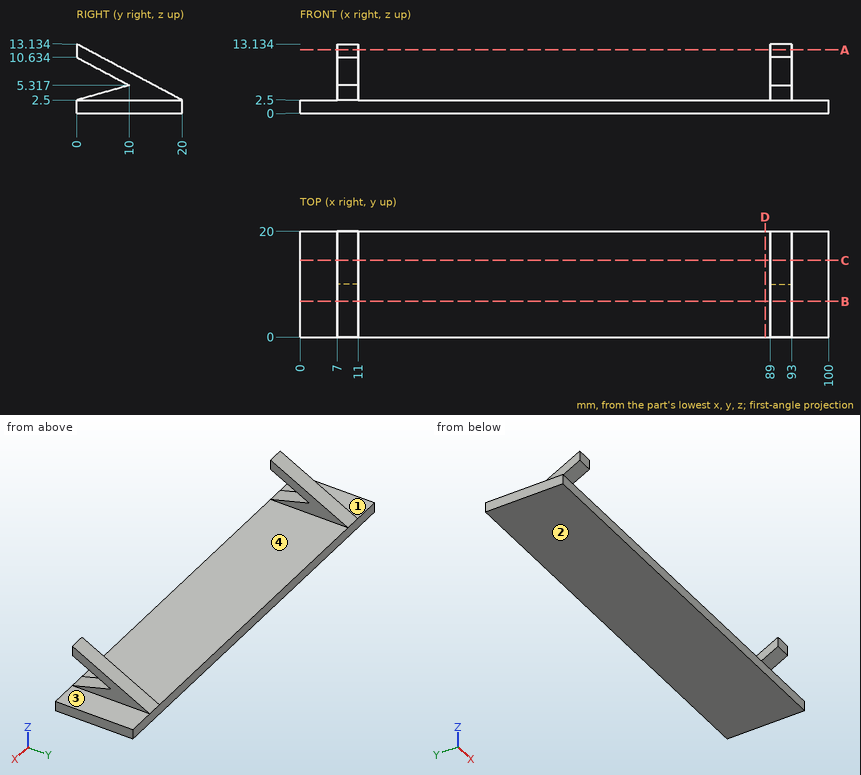
Can you work these out from the drawing? Everything is in mm from the part's minimum corner. A direction names the side the tool comes from. Round coordinates to 2 decimals unless told otherwise and drop trailing zeros. Loops run counter-clockwise (first coordinate to the right, second up) from the corner with the lowest first, then second, coordinate; pieces in that order, holes last. Notation, with made-up numbers: (-13, 42.5) - (-5, 42.5) arc R29 ccw to (-5, 70.5) - close; hole circle Ø5 at (4, 84.5). An arc over 180 degrees is marked (long way). Answer in a Markdown table with one row per item. Add a question column.
(1) If we mould it in two halves opening along X, with no side actions, what happens to the marked faces 3 and 4? For each: pulls with the +X half, pulls with the -X half, needs draft (parallel to the pull), parting line crosses it, or undercut.
(2) For the marked faces 1 and 2, which set-ups out of +Z, -Z, +X, -X, +Y, -Y let a thin tool reach every point of the face, with its end or its side?
(3) If we section it at D-D (x = 88): Please give me the cut outline in (y, z), plus the area to 3 significant figures.
(4) If we section it at C-C (y = 14.5): Please give me the cut outline in (x, z), plus the area to 3 significant figures.
(5) I'm going to push flat-ended pins straight in: pin 1 (2 mm diameter, centred on y = 10, z = 7, fed in from +X); pin 2 (6 mm diameter, centred on x = 32, y = 6, fed in from +Z); pin 3 (2 mm diameter, centred on x = 39, y = 6, fed in from -Z); pin 4 (6 mm diameter, centred on y = 10.5, z = 8.5, fed in from -X). Where does each tip first touch, or does it pass through?
(6) If we section it at B-B (y = 6.75): Please give me the cut outline in (x, z) (1 decimal), plus the area to 3 significant figures.
(7) I need wall thicknesses on line 1 along X through (y, z) = (11.25, 5); line 2 along Z through (x, y) = (14, 13.75); line 3 along Z through (x, y) = (90, 3.75). Which ranges of each line are inside material? Lowest first, please.
(8) If we section it at A-A (z = 12): Please give me the cut outline in (x, y), plus the area to 3 significant figures.
Model answer:
| question | item | result |
|---|---|---|
| 1 | face 3 | needs draft |
| 1 | face 4 | undercut |
| 2 | face 1 | +Z, -X, +Y, -Y |
| 2 | face 2 | -Z, +X, -X, +Y, -Y |
| 3 | outline | (0, 0) - (20, 0) - (20, 2.5) - (0, 2.5) - close |
| 3 | area | 50.0 mm² |
| 4 | outline | (0, 0) - (100, 0) - (100, 2.5) - (93, 2.5) - (93, 5.42) - (89, 5.42) - (89, 2.5) - (11, 2.5) - (11, 5.42) - (7, 5.42) - (7, 2.5) - (0, 2.5) - close |
| 4 | area | 273 mm² |
| 5 | pin 1 | stops at x = 93 |
| 5 | pin 2 | stops at z = 2.5 |
| 5 | pin 3 | stops at z = 0 |
| 5 | pin 4 | stops at x = 7 |
| 6 | outline | (0, 0) - (100, 0) - (100, 2.5) - (93, 2.5) - (93, 4.4) - (89, 4.4) - (89, 2.5) - (11, 2.5) - (11, 4.4) - (7, 4.4) - (7, 2.5) - (0, 2.5) - close; (7, 7) - (11, 7) - (11, 9.5) - (7, 9.5) - close; (89, 7) - (93, 7) - (93, 9.5) - (89, 9.5) - close |
| 6 | area | 285 mm² |
| 7 | line 1 | x = 7 to 11, 89 to 93 |
| 7 | line 2 | z = 0 to 2.5 |
| 7 | line 3 | z = 0 to 3.56, 8.64 to 11.14 |
| 8 | outline | (7, 0) - (11, 0) - (11, 2.13) - (7, 2.13) - close; (89, 0) - (93, 0) - (93, 2.13) - (89, 2.13) - close |
| 8 | area | 17.1 mm² |
